Part model, mm, in its own coordinate system. A direction names the side the tool comes from. Round coordinates to 2 decimals unless told otherwise and drop trailing zeros. Loops run counter-clockwise (first coordinate to the right, second up) from the corner with the lowest first, then second, coordinate; pieces in that order, holes last. Notation, with made-up numbers: M 29,86.5 L 74,86.5 A21 cw 74,107.5 Z; hole C 82,15 d5. An arc over 180 degrees is marked long. Put each result on its own line as item: value. Start each with the question number.
```python
from build123d import *
from build123d.topology import SkipClean

# Parameters (mm, degrees)
SKETCH1_W            = 36
SKETCH1_H            = 28
SKETCH1_R            = 1.25
SKETCH1_R_2          = 5.25
BOSS_EXTRUDE1_DEPTH  = 2
BOSS_EXTRUDE2_DEPTH  = 52
CUT_EXTRUDE1_DEPTH   = 2
MIRROR2_COPY_1_DEPTH = 2
CUT_EXTRUDE2_DEPTH   = 2
SKETCH6_W            = 18.304542046
SKETCH6_H            = 28
SKETCH6_R            = 3.75
SKETCH6_R_2          = 2
BOSS_EXTRUDE3_DEPTH  = 2


# Read off the part's stored shape, not the designer's step: Boss-Extrude2
with BuildPart() as part:
    # Sketch1 → Boss-Extrude1 (new body)
    with BuildSketch(Plane(origin=(0, 0, 0), x_dir=(1, 0, 0), z_dir=(0, 1, 0))):
        with Locations((11, 0)):
            Rectangle(SKETCH1_W, SKETCH1_H)
        with Locations(Location((0, 0, 0), (0, 0, 270))):
            Circle(SKETCH1_R, mode=Mode.SUBTRACT)
        with Locations(Location((22, 0, 0), (0, 0, 270))):
            Circle(SKETCH1_R, mode=Mode.SUBTRACT)
        with Locations(Location((11, 11, 0), (0, 0, 270))):
            Circle(SKETCH1_R, mode=Mode.SUBTRACT)
        with Locations(Location((11, -11, 0), (0, 0, 270))):
            Circle(SKETCH1_R, mode=Mode.SUBTRACT)
        with Locations(Location((11, 0, 0), (0, 0, 270))):
            Circle(SKETCH1_R_2, mode=Mode.SUBTRACT)
    extrude(amount=BOSS_EXTRUDE1_DEPTH)

    # Boss-Extrude2 outline → Boss-Extrude2 (add)
    with SkipClean():  # the faces are left unmerged after this step: merging them gives an invalid solid
        with BuildSketch(Plane(origin=(0, 2, 0), x_dir=(1, 0, 0), z_dir=(0, 1, 0))):
            with BuildLine():
                Line((29, 14), (-7, 14))
                Line((-7, 14), (-7, 12))
                Line((-7, 12), (10.25, 12))
                ThreePointArc((10.25, 12), (11, 12.25), (11.75, 12))
                Line((11.75, 12), (29, 12))
                Line((29, 12), (29, 14))
            make_face()
            with BuildLine():
                Line((10.25, -12), (-7, -12))
                Line((-7, -12), (-7, -14))
                Line((-7, -14), (29, -14))
                Line((29, -14), (29, -12))
                Line((29, -12), (11.75, -12))
                ThreePointArc((11.75, -12), (11, -12.25), (10.25, -12))
            make_face()
        extrude(amount=BOSS_EXTRUDE2_DEPTH)

    # Sketch5 → Cut-Extrude1 (cut)
    with SkipClean():  # the faces are left unmerged after this step: merging them gives an invalid solid
        with BuildSketch(Plane(origin=(0, 0, -14), x_dir=(-1, 0, 0), z_dir=(0, 0, -1))):
            Polygon((-29, 54), (-20.152271023, 54), (-29, 2), align=None)
        cut_extrude1 = extrude(amount=-CUT_EXTRUDE1_DEPTH, mode=Mode.SUBTRACT)

    # Mirror1: Cut-Extrude1 across plane
    with SkipClean():  # the faces are left unmerged after this step: merging them gives an invalid solid
        add(cut_extrude1.mirror(Plane(origin=(11, 0, 0), x_dir=(0, 0, 1), z_dir=(1, 0, 0))), mode=Mode.SUBTRACT)

    # Mirror2: Cut-Extrude1 across plane
    with SkipClean():  # the faces are left unmerged after this step: merging them gives an invalid solid
        add(cut_extrude1.mirror(Plane(origin=(0, 0, 0), x_dir=(1, 0, 0), z_dir=(0, 0, -1))), mode=Mode.SUBTRACT)

    # Mirror2 copy 1 sketch → Mirror2 copy 1 (cut)
    with SkipClean():  # the faces are left unmerged after this step: merging them gives an invalid solid
        with BuildSketch(Plane(origin=(22, 0, 14), x_dir=(1, 0, 0), z_dir=(0, 0, 1))):
            Polygon((-29, 54), (-20.152271023, 54), (-29, 2), align=None)
        extrude(amount=-MIRROR2_COPY_1_DEPTH, mode=Mode.SUBTRACT)

    # Sketch3 → Cut-Extrude2 (cut)
    with SkipClean():  # the faces are left unmerged after this step: merging them gives an invalid solid
        with BuildSketch(Plane(origin=(0, 0, -14), x_dir=(-1, 0, 0), z_dir=(0, 0, -1))):
            with BuildLine():
                Line((-2.889996266, 40), (-2.889996266, 12))
                ThreePointArc((-2.889996266, 12), (-11, 3.889996266), (-19.110003734, 12))
                Line((-19.110003734, 12), (-19.110003734, 40))
                ThreePointArc((-19.110003734, 40), (-11, 48.110003734), (-2.889996266, 40))
            make_face()
        cut_extrude2 = extrude(amount=-CUT_EXTRUDE2_DEPTH, mode=Mode.SUBTRACT)

    # Mirror3: Cut-Extrude2 across plane
    with SkipClean():  # the faces are left unmerged after this step: merging them gives an invalid solid
        add(cut_extrude2.mirror(Plane(origin=(0, 0, 0), x_dir=(1, 0, 0), z_dir=(0, 0, -1))), mode=Mode.SUBTRACT)

    # Sketch6 → Boss-Extrude3 (add)
    with SkipClean():  # the faces are left unmerged after this step: merging them gives an invalid solid
        with BuildSketch(Plane(origin=(0, 54, 0), x_dir=(1, 0, 0), z_dir=(0, 1, 0))):
            with Locations((11, 0)):
                Rectangle(SKETCH6_W, SKETCH6_H)
            with Locations(Location((11, 0, 0), (0, 0, 270))):
                Circle(SKETCH6_R, mode=Mode.SUBTRACT)
            with Locations(Location((11, -7.5, 0), (0, 0, 270))):
                Circle(SKETCH6_R_2, mode=Mode.SUBTRACT)
            with Locations(Location((11, 7.5, 0), (0, 0, 270))):
                Circle(SKETCH6_R_2, mode=Mode.SUBTRACT)
        extrude(amount=BOSS_EXTRUDE3_DEPTH)


solid = part.part
```
1. Drop flat-ended pins along their axis: pin 1 (2 mm diameter, centred on y = 54.5, z = -7, fed in from -X); pin 2 (5 mm diameter, centred on x = 17, z = 7, fed in from -Y); pin 3 (8 mm diameter, centred on y = 29, z = -11, fed in from -X); pin 4 (8.5 mm diameter, centred on x = 11, z = 0, fed in from -Y). Give the stop position or say it passes through.
2. Which spindle directions (+Z, -Z, +X, -X, +Y, -Y) get a long thin tool onto all of the face, cutting with end or side? Do faces 4 (the flat face through (2, 22, 12)), 5 (the flat face through (20.152, 55, 0)), 6 (the cylindrical face through (11.18, 48.11, -13.01)), 7 (the flat face through (1.848, 55, 0)). Say none if no direction does.
3. Cut at C-C, the plane z = 0. Give the cut face in (x, y), and give its area (3 significant figures).
4. Cut at D-D, the plane y = 42. Give the cut face in (x, z).
5. Cut at B-B, the plane x = 8. Give the cut face in (y, z), and give its area (3 significant figures).
6. Wall check: L1, parallel to Y at x = 3.5, z = 10.75; L2, parallel to Z at x = -1.5, y = 16; L3, parallel to X at y = 54.95, z = 0. Give the ranges that are in metal, low to high.
7. Cut at A-A, the plane z = -11. Give the cut face in (x, y), and give its area (3 significant figures).
8. Mould opens along X. For faces 1 (the flat face through (-2.514, 28.364, 13.014)), 2 (the flat face through (24.514, 28.364, -13.014)), 3 (the cylindrical face through (10.82, 3.89, -13.01)) say: released by +X, released by -X, zero draft, split by the parting line, or undercut.
Results list:
1. pin 1: stops at x = 1.85
1. pin 2: stops at y = 0
1. pin 3: stops at x = -3.06
1. pin 4: stops at y = 54
2. face 4: +X, -X
2. face 5: +Z, -Z, +X, +Y
2. face 6: +Z, -Z
2. face 7: +Z, -Z, -X, +Y
3. outline: M -7,0 L -1.25,0 L -1.25,2 L -7,2 Z; M 1.25,0 L 5.75,0 L 5.75,2 L 1.25,2 Z; M 1.85,54 L 7.25,54 L 7.25,56 L 1.85,56 Z; M 14.75,54 L 20.15,54 L 20.15,56 L 14.75,56 Z; M 16.25,0 L 20.75,0 L 20.75,2 L 16.25,2 Z; M 23.25,0 L 29,0 L 29,2 L 23.25,2 Z
3. area: 62.6 mm^2
4. outline: M -0.19,-14 L 3.14,-14 L 3.14,-12 L -0.19,-12 Z; M -0.19,12 L 3.14,12 L 3.14,14 L -0.19,14 Z; M 18.86,-14 L 22.19,-14 L 22.19,-12 L 18.86,-12 Z; M 18.86,12 L 22.19,12 L 22.19,14 L 18.86,14 Z
5. outline: M 0,-14 L 4.47,-14 L 4.47,-12 L 2,-12 L 2,-4.31 L 0,-4.31 Z; M 0,4.31 L 2,4.31 L 2,12 L 4.47,12 L 4.47,14 L 0,14 Z; M 47.53,-14 L 56,-14 L 56,-2.25 L 54,-2.25 L 54,-12 L 47.53,-12 Z; M 47.53,12 L 54,12 L 54,2.25 L 56,2.25 L 56,14 L 47.53,14 Z
5. area: 121 mm^2
6. L1: y = 0 to 2, 54 to 56
6. L2: z = -14 to -12, 12 to 14
6. L3: x = 1.85 to 7.25, 14.75 to 20.15
7. outline: M -7,0 L 9.75,0 L 9.75,2 L -7,2 Z; M 1.85,54 L 20.15,54 L 20.15,56 L 1.85,56 Z; M 12.25,0 L 29,0 L 29,2 L 12.25,2 Z
7. area: 104 mm^2
8. face 1: released by -X
8. face 2: released by +X
8. face 3: undercut
